Geometry: see drawing. Coordinates: mm, zero at the bounding-box minimum. A direction names the side the tool comes from. Give positions to 0.01 mm unless a question says otherwise; leave off trailing zeros. Loops run counter-clockwise (first coordinate to the right, second up) from the corner with the lowest first, then second, coordinate; pieces in that order, holes last. Notation, with made-up numbers: (86.25, -25) - (115.25, -25) arc R21 ccw to (115.25, -10) - close; hole circle Ø7 at (-6, 4). An arc over 180 degrees is marked (long way). Use one line per item in the form item = value.
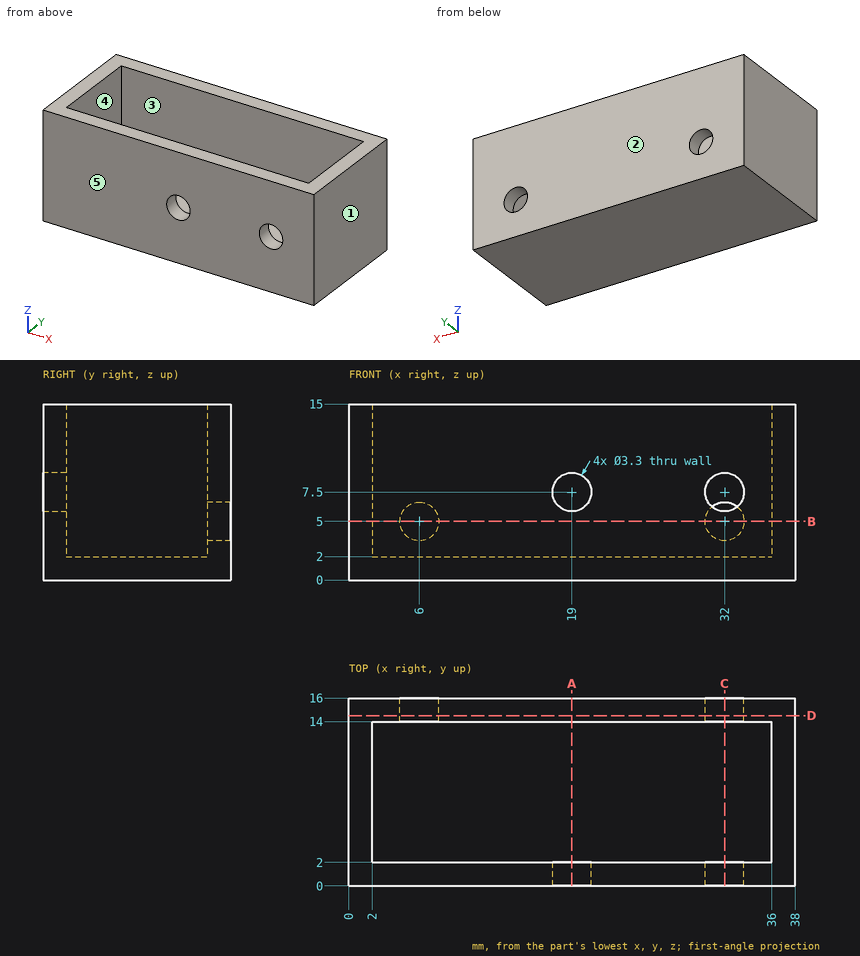
(1) Access query for the marked faces 4 and 5. Directions: +Z, -Z, +X, -X, +Y, -Y. A direction counts if a zero-diameter tool reaches every point of the face in a straight line with its end or side. Return the directions, or none.
Solution:
face_4 = +Z
face_5 = +Z, -Z, +X, -X, -Y
(2) Cut plane A-A (x = 19). Return the cut outline in (y, z).
Solution:
outline = (0, 0) - (16, 0) - (16, 15) - (14, 15) - (14, 2) - (2, 2) - (2, 5.85) - (0, 5.85) - close; (0, 9.15) - (2, 9.15) - (2, 15) - (0, 15) - close
(3) Pin query (flat end, axial travel): P1, Ø3, axis at x = 32, z = 5, coming from the +Y side; P2, Ø5, axis at x = 29.5, y = 9.5, coming from the +Z side. Return the tip coordinate at first contact, or that it passes through.
Solution:
P1 = 2
P2 = 2
(4) Cut plane B-B (z = 5). Return the cut outline in (x, y), plus the area to 3 significant figures.
Solution:
outline = (0, 0) - (38, 0) - (38, 16) - (33.65, 16) - (33.65, 14) - (36, 14) - (36, 2) - (2, 2) - (2, 14) - (4.35, 14) - (4.35, 16) - (0, 16) - close; (7.65, 14) - (30.35, 14) - (30.35, 16) - (7.65, 16) - close
area = 187 mm2
(5) Cut plane D-D (y = 14.5). Return the cut outline in (x, z), plus the area to 3 significant figures.
Solution:
outline = (0, 0) - (38, 0) - (38, 15) - (0, 15) - close; hole circle Ø3.3 at (6, 5); hole circle Ø3.3 at (32, 5)
area = 553 mm2
(6) Pull-direction query (X, two-part tool) for the marked faces 1, 2 and 3; classes: released by +X, released by -X, zero draft, split by the parting line, or undercut.
Solution:
face_1 = released by +X
face_2 = zero draft
face_3 = undercut
(7) Material intervals for L1, parallel to X at y = 15, z = 5; L2, parallel to Y at x = 25.5, z = 9; L3, parallel to X at y = 5.5, z = 6, sorted ascending. Write a range as from..to.
Solution:
L1 = 0..4.35, 7.65..30.35, 33.65..38
L2 = 0..2, 14..16
L3 = 0..2, 36..38
(8) Cut plane C-C (x = 32). Return the cut outline in (y, z).
Solution:
outline = (0, 0) - (16, 0) - (16, 3.35) - (14, 3.35) - (14, 2) - (2, 2) - (2, 5.85) - (0, 5.85) - close; (0, 9.15) - (2, 9.15) - (2, 15) - (0, 15) - close; (14, 6.65) - (16, 6.65) - (16, 15) - (14, 15) - close
